Here's the drawing with two shaded views (mm, measured from the low corner). I have some questions. A direction names the side the tool comes from. Give positions to 0.01 mm unless a question says otherwise; leave off trailing zeros. Loops run counter-clockwise (first coordinate to the right, second up) from the corner with the lowest first, then second, coordinate; pieces in that order, holes last. Notation, with made-up numbers: (-19, 21.5) - (-3, 21.5) arc R33 ccw to (-3, 56.5) - close; hole circle Ø8 at (18.25, -30.75). An arc over 180 degrees is marked (long way). Use a Markdown table: item, result. Add a question column.
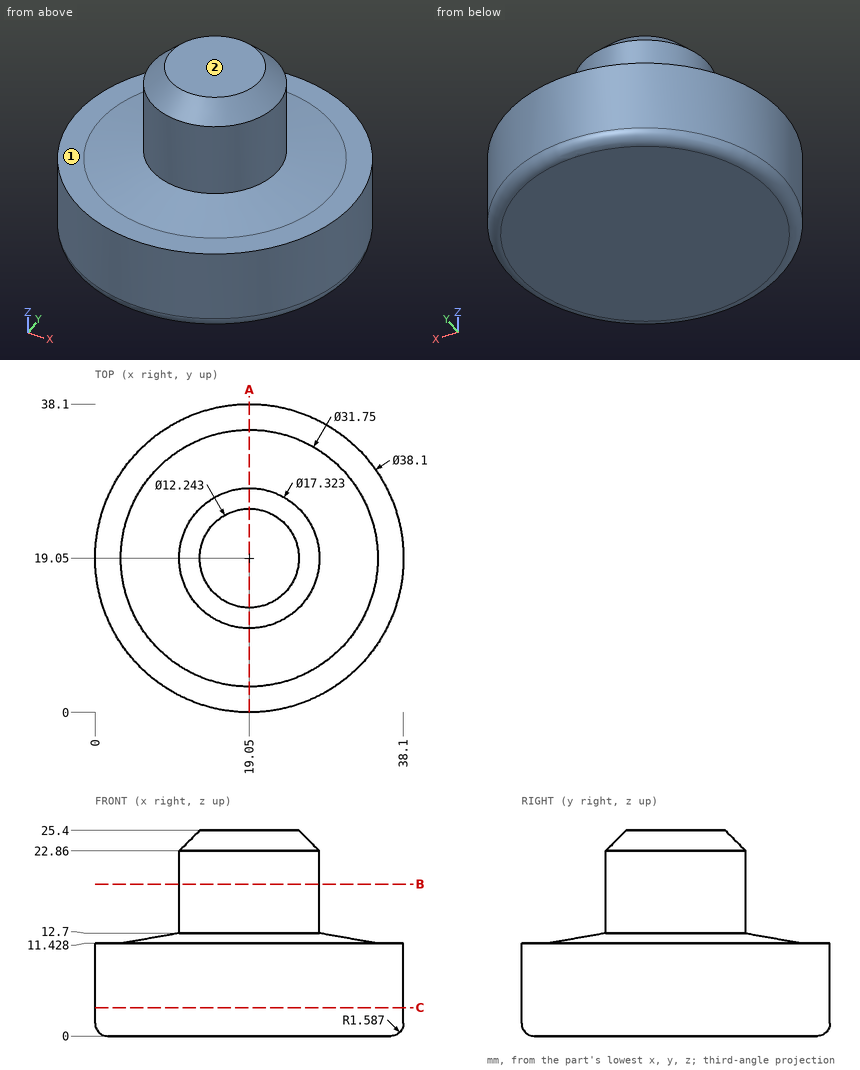
1. Suppose I cut it at C-C (z = 3.5). List the corners of the cut face in (x, y) for me.
2. Suppose I cut it at B-B (z = 18.75). List the corners of the cut face in (x, y) for me.
3. Will these pins go through, and if not, where does the flat tip stop? P1, Ø1.5, axis at x = 15, y = 13, coming from the +Z side; P2, Ø5, axis at x = 26, z = 3, coming from the -Y side; P3, Ø3, axis at x = 23.5, z = 14.5, coming from the -Y side; P4, Ø2, axis at x = 7, y = 22.5, coming from the -Z side.
4. On a 3-axis mill with a long thin cutter (end or side, diameter ignored), from which of +Z, -Z, +X, -X, +Y, -Y can I reach the whole of each face in a straight line? I mean the marked faces 1 and 2. Say none if no direction works.
5. Please list where these lines run through material, in increasing order: line 1 along Y through (x, z) = (19, 6.5); line 2 along Z through (x, y) = (11.5, 33); line 3 along X through (y, z) = (30, 11). Write a range as [from, to].
6. Suppose I cut it at A-A (x = 19.05). List the corners of the cut face in (y, z) for me (1 decimal).
Results below:
| question | item | result |
|---|---|---|
| 1 | outline | circle Ø38.1 at (19.05, 19.05) |
| 2 | outline | circle Ø17.32 at (19.05, 19.05) |
| 3 | P1 | z = 24.99 |
| 3 | P2 | y = 0.53 |
| 3 | P3 | y = 10.91 |
| 3 | P4 | z = 0 |
| 4 | face 1 | +Z |
| 4 | face 2 | +Z, +X, -X, +Y, -Y |
| 5 | line 1 | [0, 38.1] |
| 5 | line 2 | [0, 11.43] |
| 5 | line 3 | [3.46, 34.64] |
| 6 | outline | (0, 1.6) arc R1.6 ccw to (1.6, 0) - (36.5, 0) arc R1.6 ccw to (38.1, 1.6) - (38.1, 11.4) - (34.9, 11.4) - (27.7, 12.7) - (27.7, 22.9) - (25.2, 25.4) - (12.9, 25.4) - (10.4, 22.9) - (10.4, 12.7) - (3.2, 11.4) - (0, 11.4) - close |
